Work out the finished part from the listing and answer in its coordinate system (mm). A direction names the side the tool comes from. Give positions to 0.01 mm unless a question says otherwise; leave off trailing zeros. Order: outer loops, then holes, each group sorted by start corner. A loop starts at its lowest first (then second) coordinate and runs counter-clockwise, first axis right, second up. Notation, with made-up numbers: (-31.5, -7.5) - (-21.5, -7.5) arc R15 cw to (-21.5, 1.5) - close; hole circle Ø1 at (-34.75, -1.5). An arc over 180 degrees is marked (long way). Return JSON: item names as keys, results as strings. Group by question number.
from build123d import *

# Parameters (mm, degrees)
SKETCH1_R                = 2.5
BOSS_EXTRUDE1_DEPTH      = 16
BOSS_EXTRUDE2_DEPTH      = 2
BOSS_EXTRUDE2_DEPTH_BACK = 18
CHAMFER1_SIZE            = 2
FILLET1_R                = 1


with BuildPart() as part:
    # Sketch1 → Boss-Extrude1 (new body)
    with BuildSketch(Plane(origin=(0, 0, 0), x_dir=(0, 0, -1), z_dir=(1, 0, 0))):
        with BuildLine():
            Line((40, 3), (40, 17))
            Line((40, 17), (39, 18))
            Line((39, 18), (15, 18))
            Line((15, 18), (10, 18))
            Line((10, 18), (10, 19.940079597))
            ThreePointArc((10, 19.940079597), (0.884122958, 16.920488715), (-5.773502692, 10))
            Line((-5.773502692, 10), (-11.160254038, 0.669872981))
            Line((-11.160254038, 0.669872981), (-9.42820323, -0.330127019))
            Line((-9.42820323, -0.330127019), (-26.92820323, -30.641016151))
            Line((-26.92820323, -30.641016151), (-13.07179677, -38.641016151))
            Line((-13.07179677, -38.641016151), (4.42820323, -8.330127019))
            Line((4.42820323, -8.330127019), (6.160254038, -9.330127019))
            Line((6.160254038, -9.330127019), (8.660254038, -5))
            ThreePointArc((8.660254038, -5), (9.278898856, -4.055883484), (10, -3.187499614))
            Line((10, -3.187499614), (10, 2))
            Line((10, 2), (15, 2))
            Line((15, 2), (39, 2))
            Line((39, 2), (40, 3))
        make_face()
        with Locations((-15, -25.980762114)):
            Circle(SKETCH1_R, mode=Mode.SUBTRACT)
        with Locations((-7.5, -12.990381057)):
            Circle(SKETCH1_R, mode=Mode.SUBTRACT)
        with BuildLine():
            Line((19, 12.5), (36, 12.5))
            ThreePointArc((36, 12.5), (38.5, 10), (36, 7.5))
            Line((36, 7.5), (19, 7.5))
            ThreePointArc((19, 7.5), (16.5, 10), (19, 12.5))
        make_face(mode=Mode.SUBTRACT)
    extrude(amount=BOSS_EXTRUDE1_DEPTH)

    # Sketch2 → Boss-Extrude2 (add, two sides: drawn at the far end of the back side and taken through both)
    with BuildSketch(Plane(origin=(16, 0, 0), x_dir=(0, 0, -1), z_dir=(1, 0, 0)).offset(-BOSS_EXTRUDE2_DEPTH_BACK)):
        with BuildLine():
            Line((-11.160254038, 0.669872981), (6.160254038, -9.330127019))
            Line((6.160254038, -9.330127019), (8.660254038, -5))
            ThreePointArc((8.660254038, -5), (9.278898856, -4.055883484), (10, -3.187499614))
            Line((10, -3.187499614), (10, 19.940079597))
            ThreePointArc((10, 19.940079597), (0.884122958, 16.920488715), (-5.773502692, 10))
            Line((-5.773502692, 10), (-11.160254038, 0.669872981))
        make_face()
    extrude(amount=BOSS_EXTRUDE2_DEPTH + BOSS_EXTRUDE2_DEPTH_BACK)

    # Chamfer1
    chamfer1_edges = [part.edges().sort_by_distance(p)[0] for p in [
        (8, -38.641016151, 13.07179677),
        (8, -30.641016151, 26.92820323),
    ]]
    chamfer(chamfer1_edges, length=CHAMFER1_SIZE)

    # Fillet1
    fillet1_edges = [part.edges().sort_by_distance(p)[0] for p in [
        (8, 19.940079597, -10),
    ]]
    fillet(fillet1_edges, radius=FILLET1_R)


solid = part.part
1. The part is cut by section C-C (z = 16). Give the vertices of the cut face in (x, y).
2. A tool of negligible diameter and unlimited length cuts with its end or side. For faces 4 (the flat face through (0, -19, 11)), 5 (the cylindrical face through (7.9, 9.9, -16.5)), 6 (the flat face through (8, 18, -25)), 7 (the flat face through (16, -19, 11)), from which of +Z, -Z, +X, -X, +Y, -Y can it reach the whole face along a straight path? Write none if from no direction.
3. The part is cut by section B-B (x = 8.75). Give the vertices of the cut face in (y, z).
4. Consider probe 1 along X at (y, z) = (14, -17.5); probe 2 along Y at (x, z) = (3, 15); probe 3 along Y at (x, z) = (5.25, -32). Determine where each line is inside the solid, lowest interval first. Write a range as from..to.
5. Determine the mould class of faces 1 (the flat face through (8, 0, -10)), 2 (the flat face through (8, 7.5, -28)), 3 (the flat face through (7.888, -22.82, 3.937)) for opening direction Y: released by +Y, released by -Y, zero draft, split by the parting line, or undercut.
6. The part is cut by section A-A (z = -28.5). Give the vertices of the cut face in (x, y).
7. Each of these flat-tipped pins is pushed along its axis until it touches: pin 1 (5 mm diameter, centred on y = 12, z = -29.5, fed in from +X); pin 2 (5 mm diameter, centred on x = 12.5, z = -14, fed in from +Y); pin 3 (8 mm diameter, centred on x = 7.5, z = -22, fed in from -Y). Where does it stop, or does it pass through?
8. The part is cut by section D-D (y = 15). Give the vertices of the cut face in (x, z).
Answers:
{
 "1": {"outline": "(0, -36.95) - (16, -36.95) - (16, -28.27) - (0, -28.27) - close; (0, -23.69) - (16, -23.69) - (16, -11.71) - (0, -11.71) - close"},
 "2": {"face 4": "+Z, -X, -Y", "face 5": "+X, -X", "face 6": "-Z, +X, -X, +Y", "face 7": "+Z, +X, -Y"},
 "3": {"outline": "(-37.64, 14.8) - (-36.91, 12.07) - (-8.33, -4.43) - (-9.33, -6.16) - (-5, -8.66) arc R10 cw to (-3.19, -10) - (2, -10) - (2, -39) - (3, -40) - (17, -40) - (18, -39) - (18, -10) - (18.83, -10) arc R1 ccw to (19.82, -8.87) arc R20 ccw to (10, 5.77) - (0.67, 11.16) - (-0.33, 9.43) - (-28.91, 25.93) - (-31.64, 25.2) - close; hole circle Ø5 at (-25.98, 15); hole circle Ø5 at (-12.99, 7.5); hole (7.5, -36) arc R2.5 ccw to (12.5, -36) - (12.5, -19) arc R2.5 ccw to (7.5, -19) - close"},
 "4": {"probe 1": "x = 0..16", "probe 2": "y = -37.53..-28.48, -23.48..-9.98", "probe 3": "y = 2..7.5, 12.5..18"},
 "5": {"face 1": "zero draft", "face 2": "undercut", "face 3": "released by -Y"},
 "6": {"outline": "(0, 2) - (16, 2) - (16, 7.5) - (0, 7.5) - close; (0, 12.5) - (16, 12.5) - (16, 18) - (0, 18) - close"},
 "7": {"pin 1": "stops at x = 16", "pin 2": "stops at y = 18", "pin 3": "stops at y = 2"},
 "8": {"outline": "(-2, -10) - (0, -10) - (0, -40) - (16, -40) - (16, -10) - (18, -10) - (18, 1.68) - (-2, 1.68) - close"}
}
